CAD build for the part. Positions are in the model's coordinates, mm. A direction names the side the tool comes from. Give positions to 0.01 mm unless a question says otherwise; leave off trailing zeros. Write each loop counter-clockwise with the first axis right and the second up, starting at its lowest first coordinate (ties: lowest second). Pieces come first, ordered by that corner, then holes. Notation, with made-up numbers: (72.25, 51) - (90.25, 51) arc R15 cw to (90.25, 62) - close; hole circle Ø1 at (23, 2). An arc over 180 degrees is marked (long way). Write item = value, one per line. Start each with the question number.
Autodesk Inventor part; units mm, degrees
ref_plane "YZ Plane" through (0, 0, 0) normal (1, 0, 0) x (0, 1, 0)
ref_plane "XZ Plane" through (0, 0, 0) normal (0, 1, 0) x (-1, 0, 0)
ref_plane "XY Plane" through (0, 0, 0) normal (0, 0, 1) x (1, 0, 0)
sketch "Sketch1" plane through (0, 0, 0) normal (0, 1, 0) x (-1, 0, 0)
  line L0 (-21.15, 21.15) -> (21.15, 21.15)
  line L1 (21.15, 21.15) -> (21.15, -21.15)
  line L2 (21.15, -21.15) -> (-21.15, -21.15)
  line L3 (-21.15, -21.15) -> (-21.15, 21.15)
  line L4 (-21.15, 21.15) -> (21.15, -21.15) construction
  line L5 (21.15, 21.15) -> (-21.15, -21.15) construction
  circle A0 centre (0, 0) radius 3
  circle A1 centre (0, 0) radius 11
  line L6 (15.5, 15.5) -> (-15.5, 15.5)
  line L7 (-15.5, 15.5) -> (-15.5, -15.5)
  line L8 (-15.5, -15.5) -> (15.5, -15.5)
  line L9 (15.5, -15.5) -> (15.5, 15.5)
  line L10 (15.5, 15.5) -> (-15.5, -15.5) construction
  line L11 (-15.5, 15.5) -> (15.5, -15.5) construction
  dimension "d0" = 42.3
  dimension "d10" = 6
  dimension "d11" = 22
  dimension "d18" = 31
extrude "Extrusion1" add sketch "Sketch1" along normal blind 49 contours L0 L1 L2 L3 | A1 | L9 L8 L7 L6
sketch "Sketch2" plane through (-21.15, 0, -21.15) normal (-1, 0, 0) x (0, 0, 1)
  line L0 (25.6555, 40.0488) -> (16.6445, 40.0488)
  line L1 (16.6445, 40.0488) -> (16.6445, 45.3886)
  line L2 (16.6445, 45.3886) -> (25.6555, 45.3886)
  line L3 (25.6555, 45.3886) -> (25.6555, 40.0488)
  line L4 (25.6555, 40.0488) -> (16.6445, 45.3886) construction
  line L5 (16.6445, 40.0488) -> (25.6555, 45.3886) construction
  line L6 (42.3, 0) -> (0, 0)
  point P0 (21.15, 0)
  point P1 (21.15, 42.7187)
  point P2 (21.15, 40.0488)
  point P3 (21.15, 0)
extrude "Extrusion2" cut sketch "Sketch2" against normal blind 2
sketch "Sketch3" plane through (-19.15, 0, -21.15) normal (-1, 0, 0) x (0, 0, 1)
  line L0 (25.6555, 40.0488) -> (16.6445, 40.0488)
  line L1 (25.6555, 45.3886) -> (25.6555, 40.0488)
  line L2 (16.6445, 45.3886) -> (25.6555, 45.3886)
  line L3 (16.6445, 40.0488) -> (16.6445, 45.3886)
  line L4 (18.676, 42.0802) -> (23.624, 42.0802)
  line L5 (23.624, 42.0802) -> (23.624, 43.3572)
  line L6 (23.624, 43.3572) -> (18.676, 43.3572)
  line L7 (18.676, 43.3572) -> (18.676, 42.0802)
  point P0 (21.15, 0)
extrude "Extrusion3" add sketch "Sketch3" along normal blind 20 contours L7 L6 L5 L4
chamfer "Chamfer1" distance 4 angle 45 4 edges at (-21.15, 24.5, 21.15) (21.15, 24.5, 21.15) (21.15, 24.5, -21.15) (-21.15, 24.5, -21.15)
extrude "Extrusion4" add sketch "Sketch1" against normal blind 2 contours A1
sketch "Sketch4" plane through (0, 49, 0) normal (0, 1, 0) x (1, 0, 0)
  circle A0 centre (0, 0) radius 5
  circle A1 centre (0, 0) radius 4
  dimension "d14" = 10
  dimension "d15" = 1
extrude "Extrusion5" add sketch "Sketch4" along normal blind 10
hole "Hole1" at (-15.5, 0, -15.5) at (15.5, 0, -15.5) at (15.5, 0, 15.5) at (-15.5, 0, 15.5) direction (0, 1, 0) diameter 2.459 depth 8.8 tip angle 118
properties part number "L4118L1804-T6X1 — LINEAR ACTUATOR"
1. Mould opens along Z. For faces 6 (the flat face through (-19.1, 24.2, -19.2)), 7 (the cylindrical face through (-16.537, 4.462, 14.839)), 8 (the flat face through (21.15, 24, 0)) say: +Z half, -Z half, draft (parallel to the pull), parting line (faces both ways), or undercut.
2. Cut at A-A (x = 0). Give the cut face in (y, z).
3. Wall check: line 1 along Z through (x, y) = (-15.5, 2.75); line 2 along Z through (x, y) = (15, 6). Give the ranges that are in metal, low to high.
4. Tool access for faces 1 (the flat face through (-2.3, -2, -2.3)), 2 (the cylindrical face through (14.463, 4.462, 14.839)), 3 (the flat face through (-20, 45.389, 0)), 4 (the flat face through (19.2, 24.8, 19.1)), 5 (the cylindrical face through (-0.867, 53.93, -3.905)): list every direction of +Z, -Z, +X, -X, +Y, -Y with a clear straight run to the whole face (end or side of a thin tool).
5. Cut at D-D (x = -26.5). Give the cut face in (y, z), then the cut area to 3 significant figures.
6. Pin check, flat tips, straight feed: pin 1 Ø2 at (x, z) = (-15.5, -15.5) entering from -Y; pin 2 Ø5 at (x, z) = (0, 0) entering from -Y; pin 3 Ø1 at (x, y) = (-20, 42) entering from -Z; pin 4 Ø6 at (y, z) = (26.5, 7) entering from -X. Stop position of each tip, or through.
7. Cut at B-B (z = 0). Give the cut face in (x, y), then the cut area to 3 significant figures.
8. Cut at C-C (y = 47.5). Give the cut face in (x, z), then the cut area to 3 significant figures.
Output:
q1.face_6 = -Z half
q1.face_7 = undercut
q1.face_8 = draft
q2.outline = (-2, -11) - (0, -11) - (0, -21.15) - (49, -21.15) - (49, -5) - (59, -5) - (59, -4) - (49, -4) - (49, -3) - (-2, -3) - close; (-2, 3) - (49, 3) - (49, 4) - (59, 4) - (59, 5) - (49, 5) - (49, 21.15) - (0, 21.15) - (0, 11) - (-2, 11) - close
q3.line_1 = -21.15 to -16.73, -14.27 to 14.27, 16.73 to 21.15
q3.line_2 = -21.15 to -16.62, -14.38 to 14.38, 16.62 to 21.15
q4.face_1 = +Z, -Z, +X, -X, -Y
q4.face_2 = -Y
q4.face_3 = -X
q4.face_4 = +Z, +X, +Y, -Y
q4.face_5 = +Y
q5.outline = (42.08, -2.47) - (43.36, -2.47) - (43.36, 2.47) - (42.08, 2.47) - close
q5.area = 6.32 mm2
q6.pin_1 = 8.94
q6.pin_2 = through
q6.pin_3 = -18.8
q6.pin_4 = -21.15
q7.outline = (-39.15, 42.08) - (-19.15, 42.08) - (-19.15, 40.05) - (-21.15, 40.05) - (-21.15, 0) - (-11, 0) - (-11, -2) - (-3, -2) - (-3, 49) - (-4, 49) - (-4, 59) - (-5, 59) - (-5, 49) - (-21.15, 49) - (-21.15, 45.39) - (-19.15, 45.39) - (-19.15, 43.36) - (-39.15, 43.36) - close; (3, -2) - (11, -2) - (11, 0) - (21.15, 0) - (21.15, 49) - (5, 49) - (5, 59) - (4, 59) - (4, 49) - (3, 49) - close
q7.area = 1,850 mm2
q8.outline = (-21.15, -17.15) - (-17.15, -21.15) - (17.15, -21.15) - (21.15, -17.15) - (21.15, 17.15) - (17.15, 21.15) - (-17.15, 21.15) - (-21.15, 17.15) - close; hole circle Ø6 at (0, 0)
q8.area = 1,730 mm2
